Can you work these out from the model? Positions are in its coordinate system, mm. Give positions to 0.01 mm unless a question says otherwise; leave off trailing zeros. Order: outer loops, then holes, each group sorted by start corner. A loop starts at its lowest first (then second) coordinate and runs counter-clockwise, first axis right, second up. Notation, with made-up numbers: (30.5, 79.5) - (65.5, 79.5) arc R8 cw to (65.5, 84.5) - close; hole circle Ø10 at (-8, -10.75). An arc over 180 degrees is marked (long way). Answer as a JSON object with one key per item and string values.
```python
from build123d import *

# Parameters (mm, degrees)
F1_DEPTH = 8.2
F3_DEPTH = 15
F5_DEPTH = 0.6


with BuildPart() as f1:
    # F0 (on Front) → F1 (new body)
    with BuildSketch(Plane.XZ):
        with BuildLine():
            Line((1.3, 0), (0.8, 0))
            ThreePointArc((0.8, 0), (0, -0.8), (-0.8, 0))
            Line((-0.8, 0), (-1.3, 0))
            ThreePointArc((-1.3, 0), (0, -1.3), (1.3, 0))
        make_face()
    extrude(amount=F1_DEPTH)

    # F2 (on Right) → F3 (cut, symmetric)
    with BuildSketch(Plane.YZ):
        Polygon((-1.6, 0), (0, -0.4), (0, 0), align=None)
    extrude(amount=F3_DEPTH, both=True, mode=Mode.SUBTRACT)

    # F4 (on face) → F5 (join)
    with BuildSketch(Plane(origin=(0, 0, 0), x_dir=(-1, 0, 0), z_dir=(0, 1, 0))):
        with BuildLine():
            Line((0.69282, -0.4), (-0.69282, -0.4))
            ThreePointArc((-0.69282, -0.4), (0, -0.8), (0.69282, -0.4))
        make_face()
    extrude(amount=-F5_DEPTH)


solid = f1.part
```
Q1. We'd pull the mould along X, two halves only. Please class faces 1 (the face through (0, -4, -0.8)), 2 (the face through (0, -8.2, -1)), 3 (the face through (0, -4, -1.3)): released by +X, released by -X, zero draft, split by the parting line, or undercut.
Recorded:
{"face 1": "undercut", "face 2": "zero draft", "face 3": "split by the parting line"}
Q2. I need wall thicknesses on L1, parallel to X at y = -2.75, z = -0.4; L2, parallel to Z at x = -0.05, y = -7.25; L3, parallel to Z at x = 1.1, y = -3. Which ranges of each line are inside material? Lowest first, please.
Recorded:
{"L1": "x = -1.24 to -0.69, 0.69 to 1.24", "L2": "z = -1.3 to -0.8", "L3": "z = -0.69 to 0"}
Q3. If we section it at A-A, the plane x = 0: Please give me the cut outline in (y, z), then the cut area to 3 significant figures.
Recorded:
{"outline": "(-8.2, -1.3) - (0, -1.3) - (0, -0.4) - (-0.6, -0.4) - (-0.6, -0.8) - (-8.2, -0.8) - close", "area": "4.34 mm^2"}
Q4. If we section it at D-D, the plane z = -1: Please give me the cut outline in (x, y).
Recorded:
{"outline": "(-0.83, -8.2) - (0.83, -8.2) - (0.83, 0) - (-0.83, 0) - close"}
Q5. If we section it at B-B, the plane y = -2.75: Please give me the cut outline in (x, z), then the cut area to 3 significant figures.
Recorded:
{"outline": "(-1.3, 0) arc R1.3 ccw to (1.3, 0) - (0.8, 0) arc R0.8 cw to (-0.8, 0) - close", "area": "1.65 mm^2"}
Q6. If we section it at C-C, the plane x = 1.1: Please give me the cut outline in (y, z).
Recorded:
{"outline": "(-8.2, -0.69) - (0, -0.69) - (0, -0.4) - (-1.6, 0) - (-8.2, 0) - close"}
